Check sheet for the modelled part. Datum: model origin and axes. Units: mm. A direction names the side the tool comes from. Coordinates: 2 decimals unless noted, no trailing zeros. Write each loop counter-clockwise with the first axis right and the second up, starting at its lowest first coordinate (ties: lowest second). Pieces come first, ordered by that corner, then holes. Notation, with made-up numbers: M -28.75,27 L 18.25,27 A21 ccw 18.25,44 Z; hole C -33.75,-33.75 d7. An arc over 180 degrees is marked long. Answer as CSV lines item,"result". Start each with the question number.
Q1. Access from +Z, -Z, +X, -X, +Y, -Y to the whole of each face (thin tool, end or side, straight path). Record for faces 1 (the flat face through (23, 8, -15.607)), 2 (the flat face through (-3, 8, -12.661)).
Q2. Sectioned sample at B-B, the plane x = -1. Record the cut outline in (y, z).
Q3. Depth check by flat-ended pin: pin 1 Ø1.6 at (x, y) = (43, 7) entering from -Z; pin 2 Ø1.8 at (x, z) = (8.4, -12.98) entering from -Y. Enter the tip coordinate at first touch or a pass-through.
Q4. Thickness scan on line 1 along Z through (x, y) = (-3.5, 9.5); line 2 along X through (y, z) = (9, 48.5); line 3 along Z through (x, y) = (39.5, 12). Record the ranges inside material, lowest first. Write a range as from..to.
Q5. Sectioned sample at A-A, the plane y = 9.5. Record the cut outline in (x, z).
Q6. Mould release check, pull along X, two halves, no side actions. Record for faces 3 (the cylindrical face through (40.843, 8.332, 48.758)), 4 (the flat face through (40.533, 8.102, -14.32)), 5 (the flat face through (43, 8, -12.661)), 6 (the cylindrical face through (8.197, 8.332, -14.502)): pulls with the +X half, pulls with the -X half, needs draft (parallel to the pull), parting line crosses it, or undercut.
Autodesk Inventor part; units mm, degrees
ref_plane "YZ Plane" through (0, 0, 0) normal (1, 0, 0) x (0, 1, 0)
ref_plane "XZ Plane" through (0, 0, 0) normal (0, 1, 0) x (-1, 0, 0)
ref_plane "XY Plane" through (0, 0, 0) normal (0, 0, 1) x (1, 0, 0)
sketch "Sketch1" plane through (0, 0, 0) normal (0, 1, 0) x (-1, 0, 0)
  line L0 (9.5985, 62.4723) -> (-43.8177, 62.4723)
  line L1 (-43.8177, 62.4723) -> (-43.8177, -12.6609)
  line L2 (-43.8177, -12.6609) -> (9.5985, -12.6609)
  line L3 (9.5985, -12.6609) -> (9.5985, 62.4723)
  line L4 (-41.7857, -12.6609) -> (-4.3715, -12.6609)
  line L5 (-4.3715, -12.6609) -> (-4.3715, -15.6073)
  line L6 (-4.3715, -15.6073) -> (-41.7857, -15.6073)
  line L7 (-41.7857, -15.6073) -> (-41.7857, -12.6609)
  point P0 (0, 0)
  dimension "d0" = 75.1332
  dimension "d1" = 53.4162
  dimension "d2" = 37.4142
  dimension "d3" = 2.032
  dimension "d4" = 2.9464
extrude "Extrusion1" add sketch "Sketch1" along normal blind 16.4338
chamfer "Chamfer1" distance 2.54 angle 45 2 edges at (41.7857, 8.2169, -15.6073) (4.3715, 8.2169, -15.6073)
sketch "Sketch2" plane through (0, 16.4338, 0) normal (0, 1, 0) x (1, 0, 0)
  circle A0 centre (8.3974, 12.9784) radius 1.5367
  circle A1 centre (36.2866, 12.9784) radius 1.5367
  line L0 (39.2457, 15.6073) -> (6.9115, 15.6073)
  line L1 (43.8177, -62.4723) -> (43.8177, 12.6609)
  circle A2 centre (41.1761, -47.2577) radius 1.5367
  line L2 (-9.5985, -62.4723) -> (43.8177, -62.4723)
  line L3 (41.7857, 12.6609) -> (41.7857, 13.0673)
  line L4 (41.7857, 13.0673) -> (41.7857, 15.6073) construction
  line L5 (41.7857, 15.6073) -> (39.2457, 15.6073) construction
  line L6 (4.4039, 13.0673) -> (4.4039, 15.6073) construction
  line L7 (4.4039, 15.6073) -> (6.9115, 15.6073) construction
  line L8 (4.3715, 12.6609) -> (-9.5985, 12.6609) construction
  point P0 (0, 0)
  dimension "d10" = 3.0734
  dimension "d11" = 2.6289
  dimension "d12" = 3.0734
  dimension "d13" = 2.6289
  dimension "d14" = 7.5311
  dimension "d15" = 27.8892
  dimension "d16" = 15.2146
  dimension "d17" = 2.6416
  dimension "d18" = 3.0734
  dimension "d21" = 60.2361
  dimension "d22" = 4.8895
  dimension "d24" = 60.4342
  dimension "d25" = 75.1332
  dimension "d26" = 53.4162
  dimension "d27" = 2.032
  dimension "d29" = 2.9464
  dimension "d30" = 37.3818
  dimension "d31" = 2.9464
  dimension "d32" = 13.97
  dimension "d33" = 75.1332
extrude "Extrusion2" cut sketch "Sketch2" against normal blind 16.4338
equation "\"d13\" = d11"
equation "\"d18\" = d12"
properties part number "Arduino board with Sheild"
Output:
1,face 1,"-Z, +X, -X, +Y, -Y"
1,face 2,"-Z, -X, +Y, -Y"
2,outline,"M 0,-12.66 L 16.43,-12.66 L 16.43,62.47 L 0,62.47 Z"
3,pin 1,"stops at z = -12.66"
3,pin 2,"passes through"
4,line 1,"z = -12.66..62.47"
4,line 2,"x = -9.6..40.27, 42.08..43.82"
4,line 3,"z = -15.35..62.47"
5,outline,"M -9.6,-12.66 L 4.37,-12.66 L 4.37,-13.07 L 6.91,-15.61 L 39.25,-15.61 L 41.79,-13.07 L 41.79,-12.66 L 43.82,-12.66 L 43.82,62.47 L -9.6,62.47 Z; hole C 8.4,-12.98 d3.07; hole C 36.29,-12.98 d3.07; hole C 41.18,47.26 d3.07"
6,face 3,"undercut"
6,face 4,"pulls with the +X half"
6,face 5,"needs draft"
6,face 6,"undercut"
